For this review, take the finished solid that the model builds, in its own axes (mm). A direction names the side the tool comes from. Round coordinates to 2 decimals unless told otherwise and drop trailing zeros. Write each loop counter-clockwise with the first axis right and the second up, starting at its lowest first coordinate (ties: lowest second). Pieces come first, ordered by that corner, then holes. Notation, with made-up numbers: M 40.25,51 L 70.25,51 A20 ccw 70.25,67 Z; hole C 35.5,-13.5 d6. An arc over 180 degrees is marked long. Use one line per item in the form item = value. Start each with the question number.
Item 1: For line 1 (Y direction, x = -2, z = 22.25); line 2 (Y direction, x = 0, z = 12.5); line 3 (X direction, y = 13.5, z = 20.75), list the stretches that pass through material, from the lowest coordinate up. Write a range as [from, to].
Item 2: Add section B-B (x = -26). State the section outline as (y, z) points, and give its area (3 significant figures).
Item 3: Draft analysis for pull direction X (two halves, no side actions). For faces 1 (the cylindrical face through (-33.83, 18.44, 8.4)), 2 (the cylindrical face through (-20, 14, 13)), 3 (the flat face through (13, 0, 22)), state which applies: released by +X, released by -X, zero draft, split by the parting line, or undercut.
Item 4: Add section C-C (y = 14). State the section outline as (x, z) points, and give its area (3 significant figures).
Item 5: Add section D-D (x = -9). State the section outline as (y, z) points.
Item 6: For P1, Ø1.5, axis at y = 6.5, z = 13, coming from the -X side; P2, Ø2, axis at x = -39.5, y = 16, coming from the +Z side; P3, Ø1.5, axis at x = -22, z = 18.5, coming from the -Y side, all flat-tipped, find the tip position at first contact; note any pin that passes through.
Item 7: For faces 4 (the flat face through (-37, 14, 24)), 5 (the flat face through (-5.71, 20.11, 20.94)), 6 (the flat face through (-8.551, 14.826, 8.395)), list the 3-axis set-ups (+Z, -Z, +X, -X, +Y, -Y) from which the entire face can be reached by the end or side of a thin tool; tool diameter is ignored.
from build123d import *

# Parameters (mm, degrees)
EXTRUDE_1_DEPTH     = 16
EXTRUDE_2_DEPTH     = 10
CUT_EXTRUDE_1_DEPTH = 4
SKETCH_4_R          = 6
CUT_EXTRUDE_2_DEPTH = 27
CHAMFER_1_SIZE      = 1


with BuildPart() as part:
    # 草图1 → 凸台-拉伸1 (new body)
    with BuildSketch(Plane.XY):
        with BuildLine():
            Line((-30.266898407, 6.075760101), (-4.266898407, -7.924239899))
            ThreePointArc((-4.266898407, -7.924239899), (7.924239899, -4.266898407), (4.266898407, 7.924239899))
            Line((4.266898407, 7.924239899), (-21.733101593, 21.924239899))
            ThreePointArc((-21.733101593, 21.924239899), (-33.924239899, 18.266898407), (-30.266898407, 6.075760101))
        make_face()
    extrude(amount=EXTRUDE_1_DEPTH)

    # 草图2 → 凸台-拉伸2 (add)
    with BuildSketch(Plane.XY.offset(16)):
        with BuildLine():
            Line((7.111497346, 13.207066499), (-18.888502654, 27.207066499))
            ThreePointArc((-18.888502654, 27.207066499), (-39.207066499, 21.111497346), (-33.111497346, 0.792933501))
            Line((-33.111497346, 0.792933501), (-7.111497346, -13.207066499))
            ThreePointArc((-7.111497346, -13.207066499), (13.207066499, -7.111497346), (7.111497346, 13.207066499))
        make_face()
    extrude(amount=EXTRUDE_2_DEPTH)

    # 草图3 → 切除-拉伸1 (cut)
    with BuildSketch(Plane.XY.offset(26)):
        with BuildLine():
            Line((-37, 24.198039027), (-37, 3.801960973))
            ThreePointArc((-37, 3.801960973), (-41, 14), (-37, 24.198039027))
        make_face()
        with BuildLine():
            Line((11, 10.198039027), (11, -10.198039027))
            ThreePointArc((11, -10.198039027), (15, 0), (11, 10.198039027))
        make_face()
    extrude(amount=-CUT_EXTRUDE_1_DEPTH, mode=Mode.SUBTRACT)

    # 草图4 → 切除-拉伸2 (cut, through all)
    with BuildSketch(Plane(origin=(0, 0, 0), x_dir=(-1, 0, 0), z_dir=(0, 0, -1))):
        Circle(SKETCH_4_R)
        with Locations((26, 14)):
            Circle(SKETCH_4_R)
    extrude(amount=-CUT_EXTRUDE_2_DEPTH, mode=Mode.SUBTRACT)

    # 倒角1
    chamfer_1_edges = [part.edges().sort_by_distance(p)[0] for p in [
        (13.207066499, -7.111497346, 16),
        (-5.888502654, 20.207066499, 16),
        (-39.207066499, 21.111497346, 16),
        (-20.111497346, -6.207066499, 16),
        (2.45838866, -14.797172878, 26),
        (-5.888502654, 20.207066499, 26),
        (-28.45838866, 28.797172878, 26),
        (-20.111497346, -6.207066499, 26),
        (9.179877211, 11.862961451, 26),
        (-35.179877211, 2.137038549, 26),
        (-17.266898407, -0.924239899, 0),
        (6, 0, 26),
        (6, 0, 0),
        (-20, 14, 26),
        (-20, 14, 0),
        (-33.924239899, 18.266898407, 0),
        (-8.733101593, 14.924239899, 0),
        (7.924239899, -4.266898407, 0),
    ]]
    chamfer(chamfer_1_edges, length=CHAMFER_1_SIZE)


solid = part.part
Calculated:
q1.line_1 = [-14.87, -5.66], [5.66, 18.11]
q1.line_2 = [-9, -6], [6, 10.22]
q1.line_3 = [-40.99, -31.98], [-20.02, 6.57]
q2.outline = M -3.04,17 L -1.9,16 L 3.78,16 L 3.78,1 L 4.91,0 L 7,0 L 8,1 L 8,25 L 7,26 L -1.9,26 L -3.04,25 Z; M 20,1 L 21,0 L 22,0 L 23,1 L 23,16 L 28,16 L 29,17 L 29,25 L 28,26 L 21,26 L 20,25 Z
q2.area = 311 mm^2
q3.face_1 = split by the parting line
q3.face_2 = undercut
q3.face_3 = zero draft
q4.outline = M -41,17 L -40,16 L -35,16 L -35,1 L -34,0 L -33,0 L -32,1 L -32,25 L -33,26 L -37,26 L -37,22 L -41,22 Z; M -20,1 L -19,0 L -9.13,0 L -7.02,1 L -7.02,16 L 3.53,16 L 5.64,17 L 5.64,25 L 3.53,26 L -19,26 L -20,25 Z
q4.area = 580 mm^2
q5.outline = M -12.19,17 L -11.05,16 L -5.38,16 L -5.38,1 L -4.24,0 L 13.93,0 L 15.07,1 L 15.07,16 L 20.75,16 L 21.88,17 L 21.88,25 L 20.75,26 L -11.05,26 L -12.19,25 Z
q6.P1 = -31.95
q6.P2 = 22
q6.P3 = -5.59
q7.face_4 = +Z, -X, +Y, -Y
q7.face_5 = +Z, -Z, +X, +Y
q7.face_6 = -Z, +X, +Y
